Build history of the part. All positions in model axes, mm. Face numbers are marked on the shaded views. A direction names the side the tool comes from. Round coordinates to 2 decimals unless told otherwise and drop trailing zeros. Order: outer loops, then holes, each group sorted by start corner. A loop starts at its lowest first (then second) coordinate and runs counter-clockwise, first axis right, second up. Notation, with made-up numbers: (66, 6.25) -> (97, 6.25) arc R31 cw to (97, 43.25) -> close; hole circle Ø5 at (77, 89.25). An arc over 180 degrees is marked (long way). Write item = value, one per line.
from build123d import *

# Parameters (mm, degrees)
F0_R     = 5
F1_DEPTH = 60
F2_R     = 5
F3_DEPTH = 10


with BuildPart() as f1:
    # F0 (on Front) → F1 (new body)
    with BuildSketch(Plane.XZ):
        Circle(F0_R)
    extrude(amount=F1_DEPTH)

    # F2 (on face) → F3 (join)
    with BuildSketch(Plane(origin=(0, 0, 0), x_dir=(-1, 0, 0), z_dir=(0, 1, 0))):
        Polygon((5.7735026919, -10), (11.5470053838, 0), (5.7735026919, 10), (-5.7735026919, 10), (-11.5470053838, 0), (-5.7735026919, -10), align=None)
        Circle(F2_R, mode=Mode.SUBTRACT)
        Circle(F2_R)
    extrude(amount=F3_DEPTH)


solid = f1.part
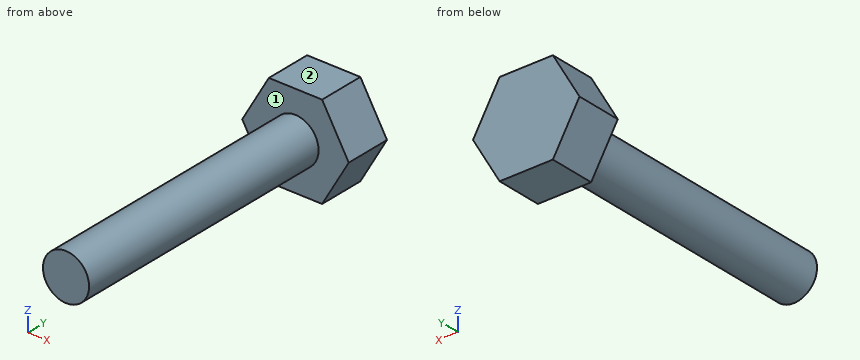
Q1. Which spindle directions (+Z, -Z, +X, -X, +Y, -Y) get a long thin tool onto all of the face, cutting with end or side? Do the marked faces 1 and 2. Say none if no direction does.
Check values:
face_1 = -Y
face_2 = +Z, +X, -X, +Y, -Y
Q2. Flat gauge pins, fed straight in: pin 1 (4 mm diameter, centred on y = -18, z = -6.5, fed in from +X); pin 2 (6 mm diameter, centred on y = -15, z = -5, fed in from +X); pin 3 (10 mm diameter, centred on x = 4, y = -36, fed in from -Z). Where does each tip first touch, or does it go through?
Check values:
pin_1 = 2.18
pin_2 = 4.58
pin_3 = -5
Q3. Cut at D-D, the plane z = -6.75. List the corners of the cut face in (x, y), and give its area (3 significant figures).
Check values:
outline = (-7.65, 0) -> (7.65, 0) -> (7.65, 10) -> (-7.65, 10) -> close
area = 153 mm²
Q4. Probe probe 1 along Y at (x, z) = (-5.75, -1); probe 2 along X at (y, z) = (-13.5, 0.25); probe 3 along X at (y, z) = (-22, -2.5). List the from-to ranges inside material, lowest first.
Check values:
probe_1 = 0 to 10
probe_2 = -4.99 to 4.99
probe_3 = -4.33 to 4.33
Q5. Cut at B-B, the plane z = -3.25. List the corners of the cut face in (x, y).
Check values:
outline = (-9.67, 0) -> (-3.8, 0) -> (-3.8, -60) -> (3.8, -60) -> (3.8, 0) -> (9.67, 0) -> (9.67, 10) -> (-9.67, 10) -> close
Q6. Cut at A-A, the plane x = 0. List the corners of the cut face in (y, z), and give its area (3 significant figures).
Check values:
outline = (-60, -5) -> (0, -5) -> (0, -10) -> (10, -10) -> (10, 10) -> (0, 10) -> (0, 5) -> (-60, 5) -> close
area = 800 mm²
Q7. Cut at C-C, the plane y = -13. List the corners of the cut face in (x, z), and give its area (3 significant figures).
Check values:
outline = circle Ø10 at (0, 0)
area = 78.5 mm²
